Read the model definition and answer for the solid it produces. Units are mm, in the model's axes. A direction names the side the tool comes from. Give positions to 0.01 mm unless a question says otherwise; leave off trailing zeros. Write each loop counter-clockwise with the first axis right and the second up, starting at its lowest first coordinate (ties: lowest second). Pieces come first, ordered by that corner, then holes. Notation, with made-up numbers: M 74.5,56.5 L 107.5,56.5 A23 ccw 107.5,67.5 Z; hole C -13.5,-33 d5. An arc over 180 degrees is marked long. Use a Markdown table: item, result. Add a question column.
Item 1: A cutting plane is placed at B-B on x = 56.25. Determine the outline of the cut face in (y, z).
Item 2: A cutting plane is placed at C-C on y = 0. Count the separate pieces of the cut face and the enclosed holes in it, then the cut area to 3 significant figures.
Item 3: Given P1, Ø10, axis at y = -3.5, z = 12.5, coming from the +X side; P2, Ø6, axis at x = -50, y = 5, coming from the +Z side; P3, Ø6, axis at y = -1.5, z = 16.5, coming from the -X side; P4, Ø2, axis at x = 56.25, y = 0, coming from the +Z side, each flat-ended and moving along its own axis, determine where each tip first touches the part or whether it passes through.
Item 4: A cutting plane is placed at A-A on z = 8.75. Determine the outline of the cut face in (x, y).
Item 5: Consider probe 1 along X at (y, z) = (-6.75, 12.75); probe 2 along Y at (x, z) = (22.05, 13); probe 3 along Y at (x, z) = (-56.25, 2.3). Determine where each line is inside the solid, lowest interval first. Write a range as [from, to].
Item 6: The mould has two halves that part along Z. Classify faces 4 (the flat face through (22, -9, 21)), 5 (the cylindrical face through (-21.579, 0.796, 10.472)), 6 (the cylindrical face through (21.621, 0.796, 10.472)), 7 (the flat face through (63.28, 7.11, 1.48)): pulls with the +Z half, pulls with the -Z half, needs draft (parallel to the pull), parting line crosses it, or undercut.
Item 7: For faces 1 (the flat face through (-20.1, -2, 11)), 2 (the flat face through (-1, 0, 0)), 3 (the flat face through (-46, 0, 3)), determine the directions among +Z, -Z, +X, -X, +Y, -Y from which every point of the face is accessible in a straight line to the end or side of a thin tool.
Item 8: A cutting plane is placed at D-D on z = 14. Determine the outline of the cut face in (x, y), then the cut area to 3 significant figures.
Autodesk Inventor part; units mm, degrees
ref_plane "YZ Plane" through (0, 0, 0) normal (1, 0, 0) x (0, 1, 0)
ref_plane "XZ Plane" through (0, 0, 0) normal (0, 1, 0) x (-1, 0, 0)
ref_plane "XY Plane" through (0, 0, 0) normal (0, 0, 1) x (1, 0, 0)
sketch "Sketch1" plane through (0, 0, 0) normal (0, 0, 1) x (1, 0, 0)
  line L0 (-56.25, 0) -> (56.25, 0) construction
  circle A0 centre (-56.25, 0) radius 1.75
  circle A1 centre (56.25, 0) radius 1.75
  line L1 (-56.25, 0) -> (56.25, 0) construction
  line L2 (-56.25, 10) -> (56.25, 10)
  line L3 (56.25, -10) -> (-56.25, -10)
  arc A2 (-56.25, 10) -> (-56.25, -10) centre (-56.25, 0) ccw
  arc A3 (56.25, -10) -> (56.25, 10) centre (56.25, 0) ccw
  line L4 (-23.1, 10) -> (-20.1, 10)
  line L5 (-20.1, 10) -> (-20.1, -10)
  line L6 (-20.1, -10) -> (-23.1, -10)
  line L7 (-23.1, -10) -> (-23.1, 10)
  line L8 (20.1, 10) -> (23.1, 10)
  line L9 (23.1, 10) -> (23.1, -10)
  line L10 (23.1, -10) -> (20.1, -10)
  line L11 (20.1, -10) -> (20.1, 10)
  line L12 (-20.1, 0) -> (20.1, 0) construction
  line L13 (0, 0) -> (0, 10) construction
  line L14 (-66.25, -4.1421) -> (-66.25, 4.1421)
  line L15 (-66.25, 4.1421) -> (-60.3921, 10)
  line L16 (-60.3921, 10) -> (-52.1079, 10)
  line L17 (-52.1079, 10) -> (-46.25, 4.1421)
  line L18 (-46.25, 4.1421) -> (-46.25, -4.1421)
  line L19 (-46.25, -4.1421) -> (-52.1079, -10)
  line L20 (-52.1079, -10) -> (-60.3921, -10)
  line L21 (-60.3921, -10) -> (-66.25, -4.1421)
  line L22 (60.3921, -10) -> (52.1079, -10)
  line L23 (52.1079, -10) -> (46.25, -4.1421)
  line L24 (46.25, -4.1421) -> (46.25, 4.1421)
  line L25 (46.25, 4.1421) -> (52.1079, 10)
  line L26 (52.1079, 10) -> (60.3921, 10)
  line L27 (60.3921, 10) -> (66.25, 4.1421)
  line L28 (66.25, 4.1421) -> (66.25, -4.1421)
  line L29 (66.25, -4.1421) -> (60.3921, -10)
  point P0 (63.3211, -7.0711)
  point P1 (66.25, 0)
  point P2 (56.25, -10)
  point P3 (63.3211, 7.0711)
  point P4 (56.25, 10)
  point P5 (-63.3211, -7.0711)
  point P6 (-66.25, 0)
  point P7 (-63.3211, 7.0711)
  dimension "d0" = 112.5
  dimension "d1" = 3.5
  dimension "d4" = 10
  dimension "d5" = 3
  dimension "d6" = 3
  dimension "d7" = 40.2
extrude "Extrusion1" add sketch "Sketch1" along normal blind 3
extrude "Extrusion2" add sketch "Sketch1" along normal blind 23 contours L2 L5 L3 L7 | L2 L9 L3 L11
sketch "Sketch2" plane through (23.1, -10, 3) normal (1, 0, 0) x (0, 0, -1)
  line L0 (0, 0) -> (-20, 20) construction
  circle A0 centre (-10, 10) radius 2.65
  point P0 (3, 10)
  dimension "d12" = 5.3
extrude "Extrusion3" cut sketch "Sketch2" against normal through all
chamfer "Chamfer1" distance 3 angle 45 6 edges at (23.1, 0, 3) (-23.1, 0, 3) (21.6, 10, 23) (21.6, -10, 23) (-21.6, -10, 23) (-21.6, 10, 23)
properties part number "soporte router"
Filled in:
| question | item | result |
|---|---|---|
| 1 | outline | M -10,0 L -1.75,0 L -1.75,3 L -10,3 Z; M 1.75,0 L 10,0 L 10,3 L 1.75,3 Z |
| 2 | separate pieces | 5 |
| 2 | enclosed holes | 0 |
| 2 | area | 474 mm² |
| 3 | P1 | x = 23.1 |
| 3 | P2 | z = 3 |
| 3 | P3 | x = -23.1 |
| 3 | P4 | through |
| 4 | outline | M -23.1,-10 L -20.1,-10 L -20.1,10 L -23.1,10 Z; M 20.1,-10 L 23.1,-10 L 23.1,10 L 20.1,10 Z |
| 5 | probe 1 | [-23.1, -20.1], [20.1, 23.1] |
| 5 | probe 2 | [-10, -2.65], [2.65, 10] |
| 5 | probe 3 | [-10, -1.75], [1.75, 10] |
| 6 | face 4 | pulls with the +Z half |
| 6 | face 5 | undercut |
| 6 | face 6 | undercut |
| 6 | face 7 | needs draft |
| 7 | face 1 | +Z, +Y, -Y |
| 7 | face 2 | -Z, +X, -X, +Y, -Y |
| 7 | face 3 | +Z, -X, +Y, -Y |
| 8 | outline | M -23.1,-10 L -20.1,-10 L -20.1,-2.45 L -23.1,-2.45 Z; M -23.1,2.45 L -20.1,2.45 L -20.1,10 L -23.1,10 Z; M 20.1,-10 L 23.1,-10 L 23.1,-2.45 L 20.1,-2.45 Z; M 20.1,2.45 L 23.1,2.45 L 23.1,10 L 20.1,10 Z |
| 8 | area | 90.6 mm² |
